The model under review builds one solid part; all positions refer to its coordinate system, in mm. Face numbers are marked on the shaded views. A direction names the side the tool comes from. Round coordinates to 2 decimals unless told otherwise and drop trailing zeros. Write each loop counter-clockwise with the first axis right and the second up, starting at its lowest first coordinate (ties: lowest second). Pieces come first, ordered by that corner, then holes. Notation, with made-up numbers: (74.25, 52) -> (117.25, 52) arc R6 ccw to (117.25, 58) -> close; hole circle Ø4 at (40.5, 46). An arc over 180 degrees is marked (long way). Answer as a JSON object with one key per item and string values. Group by question number.
1) Insertion check: pin 1 Ø3.5 at (x, z) = (0.5, 2.5) entering from +Y. The pin has a flat end and moves straight along its axis. Give the tip position at first contact, or say it passes through.
2) Machinability: for the marked faces 5, 6 and 7, which of the approach directions +Z, -Z, +X, -X, +Y, -Y give a long, thin tool a straight path to every point of the face, cutting with its end or side? Answer none if there is none.
3) We need section B-B, the plane x = -10. Write out the cut boundary in (y, z).
4) To check wall thickness, follow probe 1 along X at (y, z) = (1.7, 5); probe 2 along X at (y, z) = (4, 5); probe 3 along Z at (x, y) = (-11, 3.9). State the ranges of each line that lie inside material, in increasing order. Write a range as [from, to].
5) We need section D-D, the plane y = 0.6. Write out the cut boundary in (x, z), then the cut area to 3 significant figures.
6) We need section C-C, the plane z = -5.5. Write out the cut boundary in (x, y).
7) Mouldability with a two-part tool opening along Z and no side actions: class the marked faces 1, 2, 3 and 4 as pulls with the +Z half, pulls with the -Z half, needs draft (parallel to the pull), parting line crosses it, or undercut.
8) We need section A-A, the plane y = 3.4. Write out the cut boundary in (x, z), then the cut area to 3 significant figures.
from build123d import *

# Parameters (mm, degrees)
SKETCH1_W           = 24
SKETCH1_H           = 16
BOSS_EXTRUDE1_DEPTH = 6
SKETCH2_W           = 5
SKETCH2_H           = 6
SKETCH2_W_2         = 14
SKETCH2_H_2         = 12
CUT_EXTRUDE1_DEPTH  = 3
FILLET1_R           = 1
SKETCH3_R           = 0.889
CUT_EXTRUDE2_DEPTH  = 16.620499352


with BuildPart() as part:
    # Sketch1 → Boss-Extrude1 (new body)
    with BuildSketch(Plane(origin=(0, 0, 0), x_dir=(1, 0, 0), z_dir=(0, 1, 0))):
        Rectangle(SKETCH1_W, SKETCH1_H)
    extrude(amount=BOSS_EXTRUDE1_DEPTH)

    # Sketch2 → Cut-Extrude1 (cut)
    with BuildSketch(Plane(origin=(0, 6, 0), x_dir=(1, 0, 0), z_dir=(0, 1, 0))):
        with Locations((-9.5, 0)):
            Rectangle(SKETCH2_W, SKETCH2_H)
        Rectangle(SKETCH2_W_2, SKETCH2_H_2)
        with Locations((9.5, 0)):
            Rectangle(SKETCH2_W, SKETCH2_H)
    extrude(amount=-CUT_EXTRUDE1_DEPTH, mode=Mode.SUBTRACT)

    # Fillet1
    fillet1_edges = [part.edges().sort_by_distance(p)[0] for p in [
        (-7, 4.5, -6),
        (7, 4.5, -6),
        (7, 4.5, 6),
        (-7, 4.5, 6),
    ]]
    fillet(fillet1_edges, radius=FILLET1_R)

    # Sketch3 → Cut-Extrude2 (cut, through all)
    with BuildSketch(Plane(origin=(0, 6, 0), x_dir=(1, 0, 0), z_dir=(0, 1, 0))):
        with Locations(Location((-10, 5, 0), (0, 0, 270))):
            Circle(SKETCH3_R)
        with Locations(Location((-10, -5, 0), (0, 0, 270))):
            Circle(SKETCH3_R)
        with Locations(Location((10, -5, 0), (0, 0, 270))):
            Circle(SKETCH3_R)
        with Locations(Location((10, 5, 0), (0, 0, 270))):
            Circle(SKETCH3_R)
    extrude(amount=-CUT_EXTRUDE2_DEPTH, mode=Mode.SUBTRACT)


solid = part.part
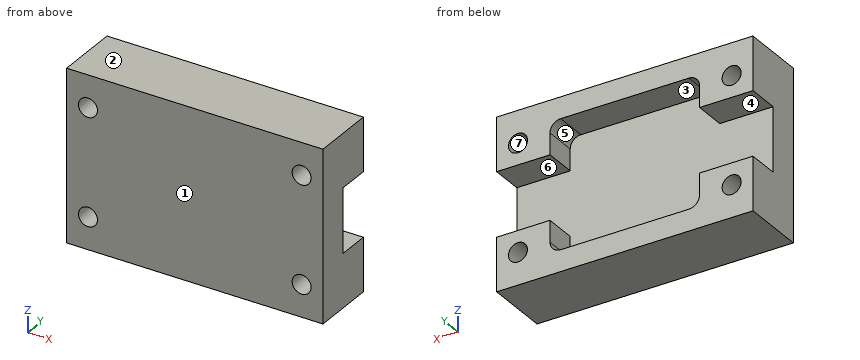
Here are the results:
{
 "1": {"pin 1": "stops at y = 3"},
 "2": {"face 5": "+Y", "face 6": "+X, -X, +Y", "face 7": "+Y, -Y"},
 "3": {"outline": "(0, -8) -> (6, -8) -> (6, -5.89) -> (0, -5.89) -> close; (0, -4.11) -> (6, -4.11) -> (6, -3) -> (3, -3) -> (3, 3) -> (6, 3) -> (6, 4.11) -> (0, 4.11) -> close; (0, 5.89) -> (6, 5.89) -> (6, 8) -> (0, 8) -> close"},
 "4": {"probe 1": "x = [-12, -10.89], [-9.11, 9.11], [10.89, 12]", "probe 2": "x = [-12, -10.89], [-9.11, -7], [7, 9.11], [10.89, 12]", "probe 3": "z = [-8, -3], [3, 8]"},
 "5": {"outline": "(-12, -8) -> (12, -8) -> (12, 8) -> (-12, 8) -> close; hole circle Ø1.78 at (-10, -5); hole circle Ø1.78 at (-10, 5); hole circle Ø1.78 at (10, -5); hole circle Ø1.78 at (10, 5)", "area": "374 mm^2"},
 "6": {"outline": "(-12, 0) -> (-10.74, 0) -> (-10.74, 6) -> (-12, 6) -> close; (-9.26, 0) -> (9.26, 0) -> (9.26, 6) -> (6.87, 6) -> (6.87, 3) -> (-6.87, 3) -> (-6.87, 6) -> (-9.26, 6) -> close; (10.74, 0) -> (12, 0) -> (12, 6) -> (10.74, 6) -> close"},
 "7": {"face 1": "needs draft", "face 2": "pulls with the +Z half", "face 3": "undercut", "face 4": "undercut"},
 "8": {"outline": "(-12, -8) -> (12, -8) -> (12, -3) -> (7, -3) -> (7, -5) arc R1 cw to (6, -6) -> (-6, -6) arc R1 cw to (-7, -5) -> (-7, -3) -> (-12, -3) -> close; (-12, 3) -> (-7, 3) -> (-7, 5) arc R1 cw to (-6, 6) -> (6, 6) arc R1 cw to (7, 5) -> (7, 3) -> (12, 3) -> (12, 8) -> (-12, 8) -> close; hole circle Ø1.78 at (-10, -5); hole circle Ø1.78 at (-10, 5); hole circle Ø1.78 at (10, -5); hole circle Ø1.78 at (10, 5)", "area": "147 mm^2"}
}
